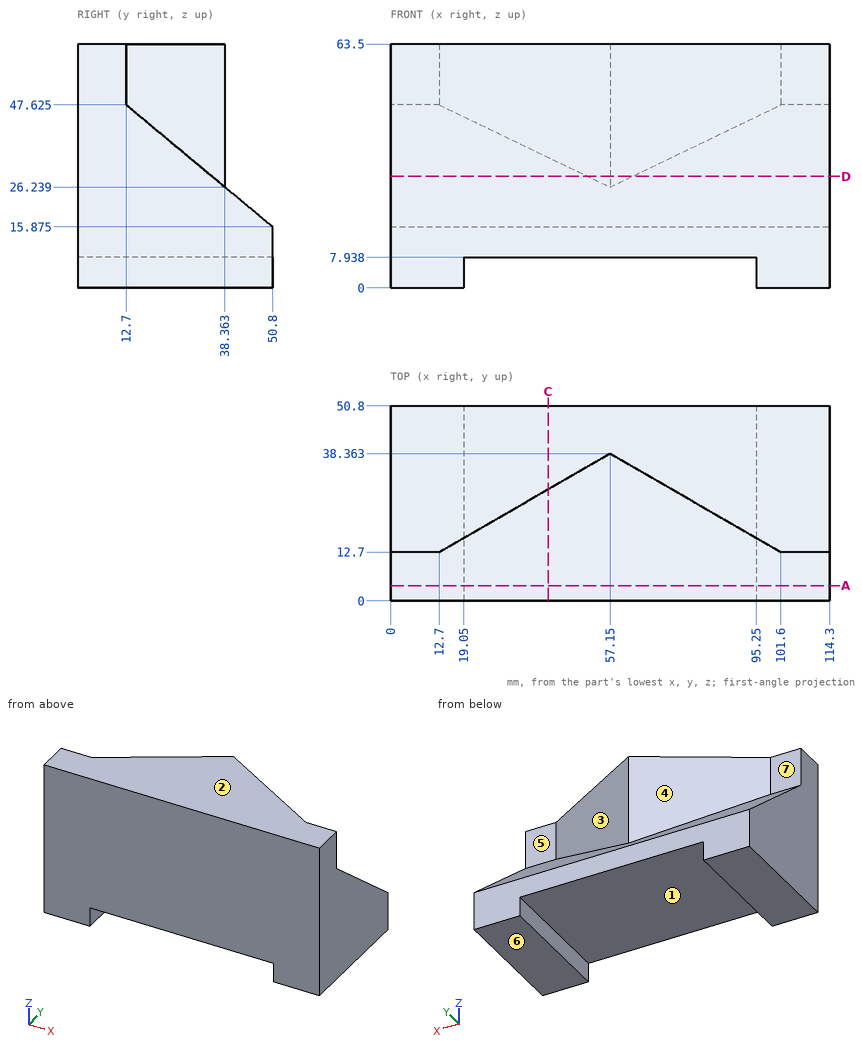
Could you check a few things on this drawing? It's one solid part, dimensions in mm from its lowest x, y, z. A direction names the side the tool comes from. Round coordinates to 2 decimals unless told otherwise and drop trailing zeros. Order: outer loops, then holes, each group sorted by start corner. A loop starts at its lowest first (then second) coordinate and runs counter-clockwise, first axis right, second up. Notation, with made-up numbers: M -22.5,-32 L 20.5,-32 A16 cw 20.5,-21 Z; hole C 48.25,30.5 d10. An arc over 180 degrees is marked long. One line per item, written item: value.
(1) Imagine slicing it at D-D (z = 29). Write out the boundary of the cut face in (x, y).
Ans:
outline: M 0,0 L 114.3,0 L 114.3,35.05 L 62.89,35.05 L 57.15,38.36 L 51.41,35.05 L 0,35.05 Z
(2) Imagine slicing it at C-C (x = 41). Write out the boundary of the cut face in (y, z) (1 decimal).
Ans:
outline: M 0,7.9 L 50.8,7.9 L 50.8,15.9 L 29,34 L 29,63.5 L 0,63.5 Z
(3) If we mould it in two halves opening along X, with no side actions, what happens to the marked faces 1, 2, 3 and 4? For each: released by +X, released by -X, zero draft, split by the parting line, or undercut.
Ans:
face 1: undercut
face 2: zero draft
face 3: released by +X
face 4: released by -X
(4) I'm going to push flat-ended pins straight in: P1, Ø1, axis at x = 85, y = 27, coming from the +Z side (1 decimal); P2, Ø2, axis at x = 51.5, z = 29.5, coming from the -Y side; P3, Ø4, axis at x = 26, y = 21, coming from the -Z side; P4, Ø14, axis at x = 108, z = 55, coming from the +Y side. Where does each tip first touch, or does it pass through?
Ans:
P1: stops at z = 36.1
P2: stops at y = 0
P3: stops at z = 7.94
P4: stops at y = 13.05
(5) I need wall thicknesses on line 1 along X through (y, z) = (36, 4); line 2 along Z through (x, y) = (21.5, 15.5); line 3 along X through (y, z) = (27.5, 38) (1 decimal). Which ranges of each line are inside material? Lowest first, please. Write a range as from..to.
Ans:
line 1: x = 0..19.05, 95.25..114.3
line 2: z = 7.94..63.5
line 3: x = 38.3..76
(6) Which directions (+Z, -Z, +X, -X, +Y, -Y) give clear straight access to the entire face, cutting with the end or side of a thin tool? Please do the marked faces 5, 6 and 7.
Ans:
face 5: +Z, +X, +Y
face 6: -Z, +X, -X, +Y, -Y
face 7: +Z, -X, +Y
(7) Imagine slicing it at A-A (y = 4). Write out the boundary of the cut face in (x, z).
Ans:
outline: M 0,0 L 19.05,0 L 19.05,7.94 L 95.25,7.94 L 95.25,0 L 114.3,0 L 114.3,63.5 L 0,63.5 Z
